Work out the finished part from the listing and answer in its coordinate system (mm). Coordinates: 2 decimals unless noted, no trailing zeros. Order: outer loops, then holes, each group sorted by start corner. A loop starts at its lowest first (then second) coordinate and runs counter-clockwise, first axis right, second up.
```python
from build123d import *

# Parameters (mm, degrees)
CROQUIS1_R              = 125
CROQUIS1_R_2            = 6
SALIENTE_EXTRUIR1_DEPTH = 20
CROQUIS2_R              = 90
SALIENTE_EXTRUIR2_DEPTH = 260


with BuildPart() as part:
    # Croquis1 → Saliente-Extruir1 (new body)
    with BuildSketch(Plane(origin=(0, 0, 0), x_dir=(0, 0, -1), z_dir=(1, 0, 0))):
        Circle(CROQUIS1_R)
        with Locations((0, -100)):
            Circle(CROQUIS1_R_2, mode=Mode.SUBTRACT)
        with Locations((-70.710678119, -70.710678119)):
            Circle(CROQUIS1_R_2, mode=Mode.SUBTRACT)
        with Locations((-100, 0)):
            Circle(CROQUIS1_R_2, mode=Mode.SUBTRACT)
        with Locations((-70.710678119, 70.710678119)):
            Circle(CROQUIS1_R_2, mode=Mode.SUBTRACT)
        with Locations((0, 100)):
            Circle(CROQUIS1_R_2, mode=Mode.SUBTRACT)
        with Locations((70.710678119, 70.710678119)):
            Circle(CROQUIS1_R_2, mode=Mode.SUBTRACT)
        with Locations((100, 0)):
            Circle(CROQUIS1_R_2, mode=Mode.SUBTRACT)
        with Locations((70.710678119, -70.710678119)):
            Circle(CROQUIS1_R_2, mode=Mode.SUBTRACT)
    extrude(amount=SALIENTE_EXTRUIR1_DEPTH)

    # Croquis2 → Saliente-Extruir2 (add)
    with BuildSketch(Plane(origin=(20, 0, 0), x_dir=(0, 0, -1), z_dir=(1, 0, 0))):
        Circle(CROQUIS2_R)
    extrude(amount=SALIENTE_EXTRUIR2_DEPTH)


solid = part.part
```
1. Consider probe 1 along Y at (x, z) = (6, 0); probe 2 along X at (y, z) = (-17.5, 97); probe 3 along Y at (x, z) = (192.5, -37). Determine where each line is inside the solid, lowest interval first.
2. The part is cut by section C-C (y = 0). Determine the outline of the cut face in (x, z), plus the area to 3 significant figures.
3. Flat-ended cylindrical pins translate along their axes: pin 1 (4 mm diameter, centred on x = 124, y = 69.5, fed in from +Z); pin 2 (5 mm diameter, centred on x = 193.5, z = 21.5, fed in from -Y); pin 3 (7 mm diameter, centred on y = -100, z = 0, fed in from +X); pin 4 (1 mm diameter, centred on y = 85, z = 48, fed in from +X). Find the tip coordinate at first contact, or state that the pin passes through.
4. The part is cut by section A-A (y = -100). Determine the outline of the cut face in (x, z).
5. The mould has two halves that part along Y. Classify faces 1 (the flat face through (20, -82, -54)), 2 (the cylindrical face through (148.18, -79.845, -41.53)), 3 (the cylindrical face through (10, 0, -94)): released by +Y, released by -Y, zero draft, split by the parting line, or undercut.
6. The part is cut by section D-D (x = 61.5). Determine the outline of the cut face in (y, z), plus the area to 3 significant figures.
Worked out:
1. probe 1: y = -125 to -106, -94 to 94, 106 to 125
1. probe 2: x = 0 to 20
1. probe 3: y = -82.04 to 82.04
2. outline: (0, -125) - (20, -125) - (20, -106) - (0, -106) - close; (0, -94) - (20, -94) - (20, -90) - (280, -90) - (280, 90) - (20, 90) - (20, 94) - (0, 94) - close; (0, 106) - (20, 106) - (20, 125) - (0, 125) - close
2. area: 51,300 mm2
3. pin 1: stops at z = 59.53
3. pin 2: stops at y = -87.97
3. pin 3: passes through
3. pin 4: stops at x = 20
4. outline: (0, -75) - (20, -75) - (20, -6) - (0, -6) - close; (0, 6) - (20, 6) - (20, 75) - (0, 75) - close
5. face 1: zero draft
5. face 2: split by the parting line
5. face 3: undercut
6. outline: circle Ø180 at (0, 0)
6. area: 25,400 mm2
